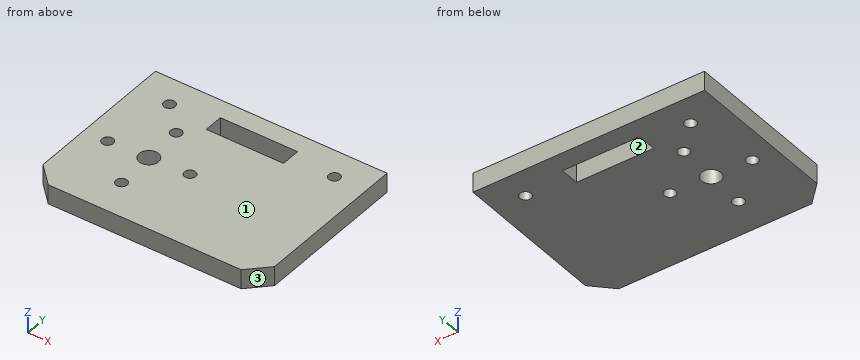
Autodesk Inventor part; units mm, degrees
ref_plane "YZ Plane" through (0, 0, 0) normal (1, 0, 0) x (0, 1, 0)
ref_plane "XZ Plane" through (0, 0, 0) normal (0, 1, 0) x (-1, 0, 0)
ref_plane "XY Plane" through (0, 0, 0) normal (0, 0, 1) x (1, 0, 0)
sketch "Sketch1" plane through (0, 0, 0) normal (0, 0, 1) x (1, 0, 0)
  line L0 (-73.2051, 41.2219) -> (-136.7051, 41.2219)
  line L1 (-143.0551, 47.5719) -> (-143.0551, 98.3719)
  line L2 (-143.0551, 98.3719) -> (-66.8551, 98.3719)
  line L3 (-66.8551, 98.3719) -> (-66.8551, 47.5719)
  line L4 (-143.0551, 47.5719) -> (-136.7051, 41.2219)
  line L5 (-73.2051, 41.2219) -> (-66.8551, 47.5719)
  point P0 (0, 0)
  point P1 (-66.8551, 41.2219)
  point P2 (-143.0551, 41.2219)
  point P3 (-117.6551, 41.2219)
  point P4 (-143.0551, 66.6219)
  point P5 (-66.8551, 72.9719)
  point P6 (-92.2551, 41.2219)
  point P7 (-143.0551, 41.2219)
  point P8 (-66.8551, 41.2219)
  dimension "d0" = 76.2
  dimension "d1" = 57.15
  dimension "d10" = 6.35
  dimension "d11" = 6.35
  dimension "d12" = 6.35
extrude "Extrusion1" add sketch "Sketch1" along normal blind 6.35
sketch "Sketch3" plane through (0, 0, 0) normal (0, 0, -1) x (-1, 0, 0)
  arc A0 (124.5928, 66.6219) -> (120.0565, 65.1716) centre (122.0928, 66.6219) ccw
  line L0 (124.5928, 66.6219) -> (120.0565, 65.1716)
  circle A1 centre (122.0928, 66.6219) radius 11
  point P0 (0, 0)
extrude "Extrusion3" [suppressed]
sketch "Sketch4" plane through (0, 0, 0) normal (0, 0, -1) x (-1, 0, 0)
  line L0 (143.0551, 92.0219) -> (133.3409, 92.0219) construction
  line L1 (143.0551, 85.6719) -> (133.3409, 85.6719) construction
  line L2 (143.0551, 85.6719) -> (143.0551, 98.3719) construction
  line L3 (35.1051, 88.8469) -> (143.0551, 88.8469) construction
  circle A0 centre (77.2251, 88.8469) radius 1.8542
  circle A1 centre (131.4867, 88.8469) radius 1.8542
  line L4 (133.3409, 92.0219) -> (133.3409, 85.6719)
  point P0 (0, 0)
  dimension "d15" = 3.7084
  dimension "d16" = 3.7084
extrude "Extrusion4" cut sketch "Sketch4" against normal through all
sketch "Sketch6" plane through (0, 0, 0) normal (0, 0, -1) x (-1, 0, 0)
  circle A0 centre (122.0928, 66.6219) radius 3.175
  circle A1 centre (108.9583, 67.1954) radius 1.8542
  circle A2 centre (122.6662, 79.7564) radius 1.8542
  circle A3 centre (135.2273, 66.0485) radius 1.8542
  circle A4 centre (121.5193, 53.4875) radius 1.8542
  circle A5 centre (122.0928, 66.6219) radius 19.05 construction
  point P0 (0, 0)
extrude "Extrusion6" cut sketch "Sketch6" against normal through all
sketch "Sketch7" plane through (0, 0, 0) normal (0, 0, -1) x (-1, 0, 0)
  line L0 (35.1051, 85.6719) -> (75.3709, 85.6719)
  line L1 (35.1051, 92.0219) -> (75.3709, 92.0219)
  line L2 (117.0559, 92.0219) -> (91.6559, 92.0219)
  line L3 (91.6559, 92.0219) -> (91.6559, 85.6719)
  line L4 (91.6559, 85.6719) -> (117.0559, 85.6719)
  line L5 (117.0559, 85.6719) -> (117.0559, 92.0219)
  line L6 (75.3709, 92.0219) -> (75.3709, 85.6719)
  line L7 (35.1051, 85.6719) -> (35.1051, 92.0219)
  point P0 (0, 0)
  dimension "d23" = 25.4
extrude "Extrusion7" cut sketch "Sketch7" against normal through all contours L5 L4 L3 L2
properties part number "projectorMountSide_RB01" material "Nylon, molybdenum disulphide"
Build history of the part. All positions in model axes, mm. Face numbers are marked on the shaded views. Round coordinates to 2 decimals unless told otherwise and drop trailing zeros. Loops run counter-clockwise (first coordinate to the right, second up) from the corner with the lowest first, then second, coordinate; pieces in that order, holes last. Notation, with made-up numbers: M 16,-15 L 26,-15 A8 ccw 26,-8 Z; hole C 54.25,34 d8. An arc over 180 degrees is marked long. Answer as CSV lines item,"result".
1. Flat gauge pin, fed straight in: P1, Ø5.5, axis at x = -122.09, y = 66.62, coming from the -Z side. Where does the tip first touch, or does it go through?
Resolved:
P1,"passes through"
2. Cut at A-A on x = -94.5. Write the cut outline in (y, z).
Resolved:
outline,"M 41.22,0 L 85.67,0 L 85.67,6.35 L 41.22,6.35 Z; M 92.02,0 L 98.37,0 L 98.37,6.35 L 92.02,6.35 Z"
3. Wall check: probe 1 along X at (y, z) = (53.5, 3.75); probe 2 along Y at (x, z) = (-100.5, 0.5); probe 3 along Y at (x, z) = (-124, 3.75). Give the ranges that are in metal, low to high. Write a range as [from, to].
Resolved:
probe 1,"x = [-143.06, -123.37], [-119.67, -66.86]"
probe 2,"y = [41.22, 85.67], [92.02, 98.37]"
probe 3,"y = [41.22, 64.08], [69.16, 78.47], [81.04, 98.37]"
4. Cut at D-D on x = -131. Write the cut outline in (y, z), then the cut area to 3 significant figures.
Resolved:
outline,"M 41.22,0 L 87.06,0 L 87.06,6.35 L 41.22,6.35 Z; M 90.64,0 L 98.37,0 L 98.37,6.35 L 90.64,6.35 Z"
area,"340 mm²"
5. Cut at C-C on y = 46. Write the cut outline in (x, z).
Resolved:
outline,"M -141.48,0 L -68.43,0 L -68.43,6.35 L -141.48,6.35 Z"
6. Cut at B-B on z = 1.5. Count the separate pieces of the cut face and the enclosed holes in it, then the cut area to 3 significant figures.
Resolved:
separate pieces,"1"
enclosed holes,"8"
area,"4,060 mm²"
7. Two-plate mould, pull along X, no slides. Class the marked faces 1, 2 and 3: released by +X, released by -X, zero draft, split by the parting line, or undercut.
Resolved:
face 1,"zero draft"
face 2,"undercut"
face 3,"released by +X"
